Design review of the part built by this model. Coordinates are the model's own, in mm. Face numbers are marked on the shaded views. A direction names the side the tool comes from. Coordinates: 2 decimals unless noted, no trailing zeros. Loops run counter-clockwise (first coordinate to the right, second up) from the corner with the lowest first, then second, coordinate; pieces in that order, holes last. Notation, with made-up numbers: (44.25, 30.5) -> (79.25, 30.5) arc R12 cw to (79.25, 43.5) -> close; hole circle Ø10 at (10.25, 24). An arc over 180 degrees is marked (long way). Answer in a Markdown table with one row per item.
```python
from build123d import *

# Parameters (mm, degrees)
SKETCH1_W             = 15
SKETCH1_H             = 30
SKETCH1_R             = 1.6
BOSS_EXTRUDE1_DEPTH   = 7
BOSS_EXTRUDE1_2_DEPTH = 7
SKETCH1_3_W           = 15
SKETCH1_3_H           = 30
BOSS_EXTRUDE2_DEPTH   = 5


with BuildPart() as part:
    # Sketch1 → Boss-Extrude1 (new body)
    with BuildSketch(Plane(origin=(0, 0, 0), x_dir=(1, 0, 0), z_dir=(0, 1, 0))):
        with Locations((-15, 0)):
            Rectangle(SKETCH1_W, SKETCH1_H)
        with Locations((-15, -7.5)):
            Circle(SKETCH1_R, mode=Mode.SUBTRACT)
        with Locations((-15, 7.5)):
            Circle(SKETCH1_R, mode=Mode.SUBTRACT)
    extrude(amount=BOSS_EXTRUDE1_DEPTH)



with BuildPart() as body_2:
    # Sketch1 → Boss-Extrude1 2 (new body)
    with BuildSketch(Plane(origin=(0, 0, 0), x_dir=(1, 0, 0), z_dir=(0, 1, 0))):
        with Locations((15, 0)):
            Rectangle(SKETCH1_W, SKETCH1_H)
        with Locations((15, -7.5)):
            Circle(SKETCH1_R, mode=Mode.SUBTRACT)
        with Locations((15, 7.5)):
            Circle(SKETCH1_R, mode=Mode.SUBTRACT)
    extrude(amount=BOSS_EXTRUDE1_2_DEPTH)


with BuildPart() as part_1:
    add(part.part)

    add(body_2.part)  # Boss-Extrude2 merges body 2
    # Sketch1<3> → Boss-Extrude2 (add)
    with BuildSketch(Plane(origin=(0, 0, 0), x_dir=(1, 0, 0), z_dir=(0, 1, 0))):
        Rectangle(SKETCH1_3_W, SKETCH1_3_H)
    extrude(amount=BOSS_EXTRUDE2_DEPTH)


solid = part_1.part
```
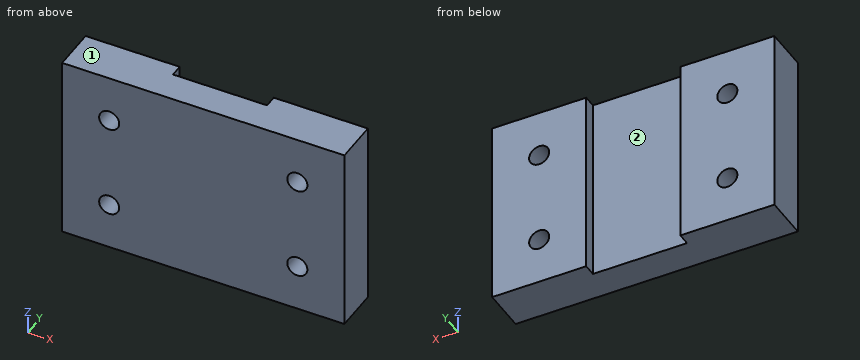
(1) For pin 1 (7.5 mm diameter, centred on x = -1.5, z = 5, fed in from +Y), flat-tipped, find the tip position at first contact; note if it passes through.
Evaluation:
| item | result |
|---|---|
| pin 1 | stops at y = 5 |
(2) Take a section at C-C on z = -7.5. Give the boundary of the cut face in (x, y).
Evaluation:
| item | result |
|---|---|
| outline | (-22.5, 0) -> (-16.6, 0) -> (-16.6, 7) -> (-22.5, 7) -> close; (-13.4, 0) -> (13.4, 0) -> (13.4, 7) -> (7.5, 7) -> (7.5, 5) -> (-7.5, 5) -> (-7.5, 7) -> (-13.4, 7) -> close; (16.6, 0) -> (22.5, 0) -> (22.5, 7) -> (16.6, 7) -> close |
(3) Take a section at D-D on y = 4. Give the boundary of the cut face in (x, z).
Evaluation:
| item | result |
|---|---|
| outline | (-22.5, -15) -> (22.5, -15) -> (22.5, 15) -> (-22.5, 15) -> close; hole circle Ø3.2 at (-15, -7.5); hole circle Ø3.2 at (-15, 7.5); hole circle Ø3.2 at (15, -7.5); hole circle Ø3.2 at (15, 7.5) |
(4) Tool access review of the marked faces 1 and 2: name each direction out of +Z, -Z, +X, -X, +Y, -Y from which nothing blocks a thin tool from reaching the whole face with its end or side.
Evaluation:
| item | result |
|---|---|
| face 1 | +Z, +X, -X, +Y, -Y |
| face 2 | +Z, -Z, +Y |
(5) Take a section at B-B on y = 6.5. Give the boundary of the cut face in (x, z).
Evaluation:
| item | result |
|---|---|
| outline | (-22.5, -15) -> (-7.5, -15) -> (-7.5, 15) -> (-22.5, 15) -> close; (7.5, -15) -> (22.5, -15) -> (22.5, 15) -> (7.5, 15) -> close; hole circle Ø3.2 at (-15, -7.5); hole circle Ø3.2 at (-15, 7.5); hole circle Ø3.2 at (15, -7.5); hole circle Ø3.2 at (15, 7.5) |
(6) Take a section at A-A on x = -15. Give the boundary of the cut face in (y, z), and give its area (3 significant figures).
Evaluation:
| item | result |
|---|---|
| outline | (0, -15) -> (7, -15) -> (7, -9.1) -> (0, -9.1) -> close; (0, -5.9) -> (7, -5.9) -> (7, 5.9) -> (0, 5.9) -> close; (0, 9.1) -> (7, 9.1) -> (7, 15) -> (0, 15) -> close |
| area | 165 mm² |
(7) To check wall thickness, follow probe 1 along Z at (x, y) = (-15, 5); probe 2 along X at (y, z) = (1.5, 7.5); probe 3 along X at (y, z) = (5.5, -7.5). State the ranges of each line that lie inside material, in increasing order.
Evaluation:
| item | result |
|---|---|
| probe 1 | z = -15 to -9.1, -5.9 to 5.9, 9.1 to 15 |
| probe 2 | x = -22.5 to -16.6, -13.4 to 13.4, 16.6 to 22.5 |
| probe 3 | x = -22.5 to -16.6, -13.4 to -7.5, 7.5 to 13.4, 16.6 to 22.5 |
